from build123d import *

# Parameters (mm, degrees)
SKETCH_1_R                       = 10
EXTRUDE_358_DEPTH                = 13
SKETCH_2_R                       = 8.5
EXTRUDE_447_DEPTH                = 5
SKETCH_3_R                       = 3
CUT_EXTRUDE_558_DEPTH            = 23.891046285
CUT_EXTRUDE_START                = -5
CUT_EXTRUDE_755_DEPTH            = 5
SKETCH_5_R                       = 1.65
CUT_EXTRUDE_910_DEPTH            = 20.209372712
FILLET_1_R                       = 1
PATTERN_CIRCULAR_1_COUNT         = 4
FILLET_1_OF_PATTERN_CIRCULAR_1_R = 1


with BuildPart() as part:
    # Эскиз1 → Extrude 358 (new body)
    with BuildSketch(Plane(origin=(0, 0, 0), x_dir=(1, 0, 0), z_dir=(0, 1, 0))):
        with Locations(Location((0, 0, 0), (0, 0, 90))):
            Circle(SKETCH_1_R)
    extrude(amount=EXTRUDE_358_DEPTH)

    # Эскиз2 → Extrude 447 (add)
    with BuildSketch(Plane(origin=(0, 13, 0), x_dir=(1, 0, 0), z_dir=(0, 1, 0))):
        with Locations(Location((0, 0, 0), (0, 0, 270))):
            Circle(SKETCH_2_R)
    extrude(amount=EXTRUDE_447_DEPTH)

    # Эскиз3 → Cut-Extrude 558 (cut, through all)
    with BuildSketch(Plane(origin=(0, 18, 0), x_dir=(1, 0, 0), z_dir=(0, 1, 0))):
        with Locations(Location((0, 0, 0), (0, 0, 270))):
            Circle(SKETCH_3_R)
    extrude(amount=-CUT_EXTRUDE_558_DEPTH, mode=Mode.SUBTRACT)

    # Эскиз4 → Cut-Extrude 755 (cut)
    with BuildSketch(Plane(origin=(0, 18, 0), x_dir=(1, 0, 0), z_dir=(0, 1, 0)).offset(CUT_EXTRUDE_START)):
        with BuildLine():
            Line((-1.65, 7), (-1.65, 8.338315178))
            ThreePointArc((-1.65, 8.338315178), (0, 8.5), (1.65, 8.338315178))
            Line((1.65, 8.338315178), (1.65, 7))
            ThreePointArc((1.65, 7), (0, 5.35), (-1.65, 7))
        make_face()
    cut_extrude_755 = extrude(amount=CUT_EXTRUDE_755_DEPTH, mode=Mode.SUBTRACT)

    # Эскиз5 → Cut-Extrude 910 (cut, through all)
    with BuildSketch(Plane(origin=(0, 13, 0), x_dir=(1, 0, 0), z_dir=(0, 1, 0))):
        with Locations(Location((0, 7, 0), (0, 0, 270))):
            Circle(SKETCH_5_R)
    cut_extrude_910 = extrude(amount=-CUT_EXTRUDE_910_DEPTH, mode=Mode.SUBTRACT)

    # Скругление1
    fillet_1_edges = [part.edges().sort_by_distance(p)[0] for p in [
        (-1.65, 15.5, -8.338315178),
        (1.65, 15.5, -8.338315178),
    ]]
    fillet(fillet_1_edges, radius=FILLET_1_R)

    # Круговой массив1: Cut-Extrude 755, Cut-Extrude 910 ×4 about axis
    pattern_circular_1_axis = Axis((0, 0, 0), (0, 1, 0))
    add([cut_extrude_755.rotate(pattern_circular_1_axis, i * 360 / PATTERN_CIRCULAR_1_COUNT) for i in range(1, PATTERN_CIRCULAR_1_COUNT)], mode=Mode.SUBTRACT)
    add([cut_extrude_910.rotate(pattern_circular_1_axis, i * 360 / PATTERN_CIRCULAR_1_COUNT) for i in range(1, PATTERN_CIRCULAR_1_COUNT)], mode=Mode.SUBTRACT)

    # Скругление1 of Круговой массив1
    fillet_1_of_pattern_circular_1_edges = [part.edges().sort_by_distance(p)[0] for p in [
        (-8.338315178, 15.5, 1.65),
        (-8.338315178, 15.5, -1.65),
        (1.65, 15.5, 8.338315178),
        (-1.65, 15.5, 8.338315178),
        (8.338315178, 15.5, -1.65),
        (8.338315178, 15.5, 1.65),
    ]]
    fillet(fillet_1_of_pattern_circular_1_edges, radius=FILLET_1_OF_PATTERN_CIRCULAR_1_R)


solid = part.part
Part model, mm, in its own coordinate system. A direction names the side the tool comes from. Coordinates: 2 decimals unless noted, no trailing zeros. Loops run counter-clockwise (first coordinate to the right, second up) from the corner with the lowest first, then second, coordinate; pieces in that order, holes last. Notation, with made-up numbers: (-5.5, 33) -> (14.5, 33) arc R13 ccw to (14.5, 45) -> close; hole circle Ø1 at (82.5, -19). An arc over 180 degrees is marked (long way). Use a Markdown table: item, result. Add a question column.
Item 1: Band-saw the part on A-A on z = 0. Write the cut outline in (x, y).
Item 2: Flat gauge pins, fed straight in: P1, Ø1, axis at y = 16, z = 3, coming from the -X side; P2, Ø3, axis at x = -2.5, y = 2.5, coming from the -Z side; P3, Ø1.5, axis at y = 6, z = -5.5, coming from the +X side. Where does each tip first touch, or does it go through?
Item 3: Pull direction Z, two halves, no side cores. Call faces 4 (the flat face through (0.1, 18, 3.5)), 5 (the cylindrical face through (5.97, 15.46, 6.05)), 6 (the cylindrical face through (2.07, 15.54, -7.83)), 7 (the cylindrical face through (-7.83, 15.54, 2.07)): +Z half, -Z half, draft (parallel to the pull), parting line (faces both ways), or undercut.
Item 4: Band-saw the part on C-C on x = 0. Write the cut outline in (y, z).
Item 5: Band-saw the part on D-D on x = -5.75. Write the cut outline in (y, z).
Item 6: Which spindle directions (+Z, -Z, +X, -X, +Y, -Y) get a long thin tool onto all of the face, cutting with end or side? Do faces 1 (the cylindrical face through (-2.07, 15.54, -7.83)), 2 (the cylindrical face through (-7.846, 15.535, -2.093)), 3 (the cylindrical face through (6.05, 15.46, -5.97)). Say none if no direction does.
Item 7: Probe probe 1 along X at (y, z) = (10.5, 0.25); probe 2 along X at (y, z) = (2.5, -1.25); probe 3 along X at (y, z) = (11.25, 7). List the from-to ranges inside material, lowest first.
Geometry says:
| question | item | result |
|---|---|---|
| 1 | outline | (-10, 0) -> (-8.65, 0) -> (-8.65, 13) -> (-10, 13) -> close; (-5.35, 0) -> (-3, 0) -> (-3, 18) -> (-5.35, 18) -> close; (3, 0) -> (5.35, 0) -> (5.35, 18) -> (3, 18) -> close; (8.65, 0) -> (10, 0) -> (10, 13) -> (8.65, 13) -> close |
| 2 | P1 | x = -8.02 |
| 2 | P2 | z = -9.95 |
| 2 | P3 | x = 8.8 |
| 3 | face 4 | draft |
| 3 | face 5 | +Z half |
| 3 | face 6 | -Z half |
| 3 | face 7 | undercut |
| 4 | outline | (0, -10) -> (13, -10) -> (13, -8.65) -> (0, -8.65) -> close; (0, -5.35) -> (18, -5.35) -> (18, -3) -> (0, -3) -> close; (0, 3) -> (18, 3) -> (18, 5.35) -> (0, 5.35) -> close; (0, 8.65) -> (13, 8.65) -> (13, 10) -> (0, 10) -> close |
| 5 | outline | (0, -8.18) -> (13, -8.18) -> (13, -6.26) -> (18, -6.26) -> (18, -1.08) -> (0, -1.08) -> close; (0, 1.08) -> (18, 1.08) -> (18, 6.26) -> (13, 6.26) -> (13, 8.18) -> (0, 8.18) -> close |
| 6 | face 1 | -Z, +Y |
| 6 | face 2 | -X, +Y |
| 6 | face 3 | -Z, +X, +Y |
| 7 | probe 1 | -10 to -8.63, -5.37 to -2.99, 2.99 to 5.37, 8.63 to 10 |
| 7 | probe 2 | -9.92 to -8.08, -5.92 to -2.73, 2.73 to 5.92, 8.08 to 9.92 |
| 7 | probe 3 | -7.14 to -1.65, 1.65 to 7.14 |
